Build history of the part. All positions in model axes, mm. Round coordinates to 2 decimals unless told otherwise and drop trailing zeros. Write each loop counter-clockwise with the first axis right and the second up, starting at its lowest first coordinate (ties: lowest second). Pieces come first, ordered by that corner, then holes. Notation, with made-up numbers: (83, 18.5) - (141, 18.5) arc R23 ccw to (141, 37.5) - close; hole circle Ø10 at (-34, -13). An arc over 180 degrees is marked (long way). Write each question's results on one line, items separated by ' | '.
from build123d import *

# Parameters (mm, degrees)
F0_R     = 7
F0_R_2   = 5
F1_DEPTH = 15
F2_SIZE2 = 0.2886751346
F2_SIZE  = 0.5
F3_SIZE2 = 0.2886751346
F3_SIZE  = 0.5


with BuildPart() as f1:
    # F0 (on Top) → F1 (new body)
    with BuildSketch(Plane.XY):
        Circle(F0_R)
        Circle(F0_R_2, mode=Mode.SUBTRACT)
    extrude(amount=F1_DEPTH)

    # F2
    f2_edges = [f1.edges().sort_by_distance(p)[0] for p in [
        (-7, 0, 15),
    ]]
    f2_side = f1.faces().sort_by_distance((-7, 0, 7.5))[0]
    chamfer(f2_edges, length=F2_SIZE, length2=F2_SIZE2, reference=f2_side)

    # F3
    f3_edges = [f1.edges().sort_by_distance(p)[0] for p in [
        (-5, 0, 0),
    ]]
    f3_side = f1.faces().sort_by_distance((-5, 0, 7.5))[0]
    chamfer(f3_edges, length=F3_SIZE, length2=F3_SIZE2, reference=f3_side)


solid = f1.part
(1) Drill centre lines: probe 1 along Y at (x, z) = (0, 11.75); probe 2 along X at (y, z) = (-4.25, 13); probe 3 along X at (y, z) = (1, 10). Where is each one in solid material? Low to high. Write a range as [from, to].
Worked answers:
probe 1: y = [-7, -5], [5, 7] | probe 2: x = [-5.56, -2.63], [2.63, 5.56] | probe 3: x = [-6.93, -4.9], [4.9, 6.93]
(2) Slice it at A-A, the plane x = 0. Write the cut outline in (y, z), and give its area (3 significant figures).
Worked answers:
outline: (-7, 0) - (-5.29, 0) - (-5, 0.5) - (-5, 15) - (-6.71, 15) - (-7, 14.5) - close; (5, 0.5) - (5.29, 0) - (7, 0) - (7, 14.5) - (6.71, 15) - (5, 15) - close | area: 59.7 mm2
(3) Two-plate mould, pull along Y, no slides. Class faces 1 (the flat face through (-5, -2, 15)), 2 (the cylindrical face through (-1.08, -4.88, 7.65)), 3 (the cylindrical face through (6.466, -2.681, 7.148)): released by +Y, released by -Y, zero draft, split by the parting line, or undercut.
Worked answers:
face 1: zero draft | face 2: undercut | face 3: split by the parting line
(4) Flat gauge pins, fed straight in: pin 1 Ø3 at (x, z) = (5.5, 2.5) entering from -Y; pin 2 Ø5 at (x, z) = (0.5, 3) entering from -Y; pin 3 Ø1.5 at (x, z) = (2.5, 8) entering from +Y; pin 4 Ø1.5 at (y, z) = (-2, 5.5) entering from -X. Where does each tip first touch, or does it go through?
Worked answers:
pin 1: stops at y = -5.74 | pin 2: stops at y = -7 | pin 3: stops at y = 6.78 | pin 4: stops at x = -6.89
